For this review, take the finished solid that the model builds, in its own axes (mm). A direction names the side the tool comes from. Round coordinates to 2 decimals unless told otherwise and drop trailing zeros. Write each loop counter-clockwise with the first axis right and the second up, starting at its lowest first coordinate (ties: lowest second). Pieces come first, ordered by that corner, then holes.
from build123d import *

# Parameters (mm, degrees)
F1_DEPTH = 6.35
F2_R     = 3.175
F3_DEPTH = 9.525
F4_R     = 3.175
F5_DEPTH = 9.525
F6_R     = 3.175
F7_DEPTH = 12.7


with BuildPart() as f1:
    # F0 (on Right) → F1 (new body, symmetric)
    with BuildSketch(Plane.YZ):
        with BuildLine():
            Line((-6.519195886, -6.223), (6.519195886, -6.223))
            ThreePointArc((6.519195886, -6.223), (0, 13.462), (-6.519195886, -6.223))
        make_face()
    extrude(amount=F1_DEPTH, both=True)



with BuildPart() as f3:
    # F2 (on Right) → F3 (new body, symmetric)
    with BuildSketch(Plane.YZ):
        Circle(F2_R)
    extrude(amount=F3_DEPTH, both=True)


with BuildPart() as f1_1:
    add(f1.part)

    add(f3.part)  # F5 merges F3
    # F4 (on Right) → F5 (join, symmetric)
    with BuildSketch(Plane.YZ):
        Circle(F4_R)
    extrude(amount=F5_DEPTH, both=True)

    # F6 (on face) → F7 (cut)
    with BuildSketch(Plane(origin=(0, 0, -6.223), x_dir=(1, 0, 0), z_dir=(0, 0, -1))):
        Circle(F6_R)
    extrude(amount=-F7_DEPTH, mode=Mode.SUBTRACT)


solid = f1_1.part
(1) Mouldability with a two-part tool opening along X and no side actions: class faces 1 (the face through (-6.35, 0, 4)), 2 (the face through (6.35, 0, 4)), 3 (the face through (-0.69, 3.1, 0.04)) as pulls with the +X half, pulls with the -X half, needs draft (parallel to the pull), parting line crosses it, or undercut.
Geometry check:
face 1: pulls with the -X half
face 2: pulls with the +X half
face 3: undercut
(2) For line 1 along X through (y, z) = (0, -1) (3 decimals); line 2 along Y through (x, z) = (0, 0) (3 decimals); line 3 along X through (y, z) = (1.25, 12.5), list the stretches that pass through material, from the lowest coordinate up.
Geometry check:
line 1: x = -9.525 to -3.175, 3.175 to 9.525
line 2: y = -10.623 to -3.175, 3.175 to 10.623
line 3: x = -6.35 to 6.35
(3) We need section A-A, the plane z = 2.5. Give the boundary of the cut face in (x, y) (3 decimals).
Geometry check:
outline: (-9.525, -1.957) - (-6.35, -1.957) - (-6.35, -10.922) - (6.35, -10.922) - (6.35, -1.957) - (9.525, -1.957) - (9.525, 1.957) - (6.35, 1.957) - (6.35, 10.922) - (-6.35, 10.922) - (-6.35, 1.957) - (-9.525, 1.957) - close; hole circle Ø6.35 at (0, 0)
(4) We need section D-D, the plane z = 0. Give the boundary of the cut face in (x, y) (3 decimals).
Geometry check:
outline: (-9.525, -3.175) - (-6.35, -3.175) - (-6.35, -10.623) - (6.35, -10.623) - (6.35, -3.175) - (9.525, -3.175) - (9.525, 3.175) - (6.35, 3.175) - (6.35, 10.623) - (-6.35, 10.623) - (-6.35, 3.175) - (-9.525, 3.175) - close; hole circle Ø6.35 at (0, 0)
(5) We need section C-C, the plane y = 2. Give the boundary of the cut face in (x, z) (3 decimals), and give its area (3 significant figures).
Geometry check:
outline: (-9.525, -2.466) - (-6.35, -2.466) - (-6.35, -6.223) - (-2.466, -6.223) - (-2.466, 6.477) - (2.466, 6.477) - (2.466, -6.223) - (6.35, -6.223) - (6.35, -2.466) - (9.525, -2.466) - (9.525, 2.466) - (6.35, 2.466) - (6.35, 13.277) - (-6.35, 13.277) - (-6.35, 2.466) - (-9.525, 2.466) - close
area: 216 mm2
(6) We need section B-B, the plane x = 0. Give the boundary of the cut face in (y, z) (3 decimals), and give its area (3 significant figures).
Geometry check:
outline: (-6.519, -6.223) - (-3.175, -6.223) - (-3.175, 6.477) - (3.175, 6.477) - (3.175, -6.223) - (6.519, -6.223) arc R10.922 ccw (long way) to start
area: 275 mm2
(7) For pin 1 Ø3 at (y, z) = (4, 5) entering from +X; pin 2 Ø5 at (x, y) = (0, 0.5) entering from -Z; pin 3 Ø1 at (x, z) = (3, -3.5) entering from -Y, all flat-tipped, find the tip position at first contact; note any pin that passes through.
Geometry check:
pin 1: stops at x = 6.35
pin 2: stops at z = 6.48
pin 3: stops at y = -9.41
(8) For faces 4 (the face through (7.96, -0.69, -3.1)), 5 (the face through (0, 0, 6.477)), 6 (the face through (-7.92, -0.69, -3.1)), list the 3-axis set-ups (+Z, -Z, +X, -X, +Y, -Y) from which the entire face can be reached by the end or side of a thin tool; tool diameter is ignored.
Geometry check:
face 4: +X
face 5: -Z
face 6: -X
